For this review, take the finished solid that the model builds, in its own axes (mm). A direction names the side the tool comes from. Coordinates: 2 decimals unless noted, no trailing zeros. Loops run counter-clockwise (first coordinate to the right, second up) from the corner with the lowest first, then second, coordinate; pieces in that order, holes last. Notation, with made-up numbers: M -13.5,25.25 L -4.5,25.25 A9 ccw -4.5,31.25 Z; hole C 70.25,-22.5 d6. An arc over 180 degrees is marked long. Write item = value, one per line.
from build123d import *

# Parameters (mm, degrees)
IZIM3_W                     = 4
IZIM3_H                     = 1
Y_KSEKLIK_EKSTR_ZYON1_DEPTH = 1
DAIRESEL_KAPLAMA1_COUNT     = 6


with BuildPart() as part:
    # izim1 → D_nd_r2 (revolve)
    with BuildSketch(Plane.XY, mode=Mode.PRIVATE) as d_nd_r2_sk:
        Polygon((-44.562063093, 33.737210457), (-44.562063093, 31.737210457), (-33.555064496, 31.737210457), (0, 35), (0, 36), (15, 36), (15, 38), (0, 38), (0, 40), align=None)
    revolve(d_nd_r2_sk.sketch.rotate(Axis((-44.316348886, 0, 0), (1, 0, 0)), 90), axis=Axis((-44.316348886, 0, 0), (1, 0, 0)))

    # izim3 → Y_kseklik-Ekstr_zyon1 (add, symmetric)
    with BuildSketch(Plane(origin=(0, 0, 0), x_dir=(1, 0, 0), z_dir=(0, 1, 0))):
        with Locations((2, -35.5)):
            Rectangle(IZIM3_W, IZIM3_H)
    y_kseklik_ekstr_zyon1 = extrude(amount=Y_KSEKLIK_EKSTR_ZYON1_DEPTH, both=True)

    # Dairesel Kaplama1: Y_kseklik-Ekstr_zyon1 ×6 about axis
    dairesel_kaplama1_axis = Axis((0, 0, 0), (1, 0, 0))
    for i in range(1, DAIRESEL_KAPLAMA1_COUNT):
        add(y_kseklik_ekstr_zyon1.rotate(dairesel_kaplama1_axis, i * 360 / DAIRESEL_KAPLAMA1_COUNT))


solid = part.part
Q1. Add section C-C (x = -6). Write out the cut boundary in (y, z), and give its area (3 significant figures).
Solved:
outline = C 0,0 d78.31; hole C 0,0 d68.83
area = 1,100 mm²
Q2. Add section B-B (x = -16). Write out the cut boundary in (y, z), and give its area (3 significant figures).
Solved:
outline = C 0,0 d75.5; hole C 0,0 d66.89
area = 963 mm²
Q3. For pin 1 Ø0.5 at (x, z) = (1.5, -35.5) entering from +Y; pin 2 Ø0.6 at (y, z) = (30.5, -17.5) entering from +X; pin 3 Ø10 at (x, z) = (-9, 30) entering from +Y, all flat-tipped, find the tip position at first contact; note any pin that passes through.
Solved:
pin_1 = 14.19
pin_2 = 4
pin_3 = 29.69
Q4. Machinability: for faces 4 (the face through (2, 0, 35)), 5 (the face through (-44.562, 20, 25)), which of the approach directions +Z, -Z, +X, -X, +Y, -Y give a long, thin tool a straight path to every point of the face, cutting with its end or side? Answer none if there is none.
Solved:
face_4 = +X
face_5 = +Z, -Z, -X, +Y, -Y
Q5. Draft analysis for pull direction Z (two halves, no side actions). For faces 1 (the face through (-27.54, -10.85, 34.46)), 2 (the face through (15, 28, 23)), 3 (the face through (0, -17, 31)), state which applies: +Z half, -Z half, draft (parallel to the pull), parting line (faces both ways), or undercut.
Solved:
face_1 = parting line
face_2 = draft
face_3 = undercut
Q6. For line 1 along Y through (x, z) = (11.75, 0); line 2 along Z through (x, y) = (-21, 3.5); line 3 along Y through (x, z) = (-37, 2), list the stretches that pass through material, from the lowest coordinate up.
Solved:
line_1 = -38 to -36, 36 to 38
line_2 = -36.88 to -32.77, 32.77 to 36.88
line_3 = -34.74 to -31.67, 31.67 to 34.74
Q7. Add section A-A (z = 0). Write out the cut boundary in (x, y).
Solved:
outline = M -44.56,-33.74 L 0,-40 L 0,-38 L 15,-38 L 15,-36 L 0,-36 L 0,-35 L -33.56,-31.74 L -44.56,-31.74 Z; M -44.56,31.74 L -33.56,31.74 L 0,35 L 0,36 L 15,36 L 15,38 L 0,38 L 0,40 L -44.56,33.74 Z
